from build123d import *

# Parameters (mm, degrees)
SKETCH_190_W        = 36
SKETCH_190_H        = 26.8
EXTRUDE_1_DEPTH     = 16.5
SKETCH_353_W        = 34
SKETCH_353_H        = 24.8
CUT_EXTRUDE_1_DEPTH = 14.5
SKETCH_4_W          = 23.5
SKETCH_4_H          = 23.5
CUT_EXTRUDE_2_DEPTH = 1
SKETCH_5_R          = 11.7
CUT_EXTRUDE_3_DEPTH = 6
SKETCH_11_W         = 2.5
SKETCH_11_H         = 1
CUT_EXTRUDE_6_DEPTH = 2


with BuildPart() as part:
    # Sketch 190 → 凸台-拉伸1 (new body)
    with BuildSketch(Plane(origin=(0, 0, 0), x_dir=(1, 0, 0), z_dir=(0, 1, 0))):
        Rectangle(SKETCH_190_W, SKETCH_190_H)
    extrude(amount=EXTRUDE_1_DEPTH)

    # Sketch 353 → 切除-拉伸1 (cut)
    with BuildSketch(Plane(origin=(0, 0, 0), x_dir=(-1, 0, 0), z_dir=(0, -1, 0))):
        Rectangle(SKETCH_353_W, SKETCH_353_H)
    extrude(amount=-CUT_EXTRUDE_1_DEPTH, mode=Mode.SUBTRACT)

    # 草图4 → 切除-拉伸2 (cut)
    with BuildSketch(Plane.XZ.offset(-14.5)):
        Rectangle(SKETCH_4_W, SKETCH_4_H)
    extrude(amount=-CUT_EXTRUDE_2_DEPTH, mode=Mode.SUBTRACT)

    # 草图5 → 切除-拉伸3 (cut)
    with BuildSketch(Plane.XZ.offset(-15.5)):
        Circle(SKETCH_5_R)
    extrude(amount=-CUT_EXTRUDE_3_DEPTH, mode=Mode.SUBTRACT)

    # 草图11 → 切除-拉伸6 (cut)
    with BuildSketch(Plane(origin=(0, 0, 0), x_dir=(-1, 0, 0), z_dir=(0, -1, 0))):
        with Locations((0, -12.9)):
            Rectangle(SKETCH_11_W, SKETCH_11_H)
    extrude(amount=-CUT_EXTRUDE_6_DEPTH, mode=Mode.SUBTRACT)


solid = part.part
Design review of the part built by this model. Coordinates are the model's own, in mm. A direction names the side the tool comes from. Give positions to 0.01 mm unless a question says otherwise; leave off trailing zeros. Order: outer loops, then holes, each group sorted by start corner. A loop starts at its lowest first (then second) coordinate and runs counter-clockwise, first axis right, second up. Notation, with made-up numbers: (14, -4) - (44, -4) arc R22 cw to (44, 19) - close; hole circle Ø9 at (30.5, -34.75). An arc over 180 degrees is marked (long way). Use CSV: the item, a comma, the result in double quotes. Start each with the question number.
Q1. For line 1 (Z direction, x = 0, y = 16.1); line 2 (X direction, y = 13.5, z = -7.5); line 3 (Z direction, x = -5.5, y = 3.25), list the stretches that pass through material, from the lowest coordinate up.
Q2. Take a section at C-C (y = 2.75). State the section outline as (x, z) points.
Q3. Take a section at A-A (x = 0). State the section outline as (y, z) points.
Q4. Machinability: for faces 4 (the face through (0, 15, -11.75)), 5 (the face through (-1.25, 1, 13)), 6 (the face through (0, 16.5, -12)), which of the approach directions +Z, -Z, +X, -X, +Y, -Y give a long, thin tool a straight path to every point of the face, cutting with its end or side? Answer none if there is none.
Q5. Take a section at B-B (z = 0). State the section outline as (x, y) points, and give its area (3 significant figures).
Q6. Take a section at D-D (x = 13). State the section outline as (y, z) points.
Q7. Draft analysis for pull direction X (two halves, no side actions). For faces 1 (the face through (0, 0, -13)), 2 (the face through (18, 8, 0)), 3 (the face through (0, 2, 13)), state which applies: pulls with the +X half, pulls with the -X half, needs draft (parallel to the pull), parting line crosses it, or undercut.
Q8. For P1, Ø1.5, axis at x = -13, z = 4.5, coming from the -Y side; P2, Ø5, axis at x = 6.5, z = -3.5, coming from the -Y side, all flat-tipped, find the tip position at first contact; note any pin that passes through.
Calculated:
1,line 1,"z = -13.4 to -11.7, 11.7 to 13.4"
1,line 2,"x = -18 to -17, 17 to 18"
1,line 3,"z = -13.4 to -12.4, 12.4 to 13.4"
2,outline,"(-18, -13.4) - (18, -13.4) - (18, 13.4) - (-18, 13.4) - close; hole (-17, -12.4) - (17, -12.4) - (17, 12.4) - (-17, 12.4) - close"
3,outline,"(0, -13.4) - (16.5, -13.4) - (16.5, -11.7) - (15.5, -11.7) - (15.5, -11.75) - (14.5, -11.75) - (14.5, -12.4) - (0, -12.4) - close; (2, 12.4) - (14.5, 12.4) - (14.5, 11.75) - (15.5, 11.75) - (15.5, 11.7) - (16.5, 11.7) - (16.5, 13.4) - (2, 13.4) - close"
4,face 4,"-Y"
4,face 5,"+Z, -Y"
4,face 6,"+Z, -Z, +X, -X, +Y"
5,outline,"(-18, 0) - (-17, 0) - (-17, 14.5) - (-11.75, 14.5) - (-11.75, 15.5) - (-11.7, 15.5) - (-11.7, 16.5) - (-18, 16.5) - close; (11.7, 15.5) - (11.75, 15.5) - (11.75, 14.5) - (17, 14.5) - (17, 0) - (18, 0) - (18, 16.5) - (11.7, 16.5) - close"
5,area,"54.1 mm²"
6,outline,"(0, -13.4) - (16.5, -13.4) - (16.5, 13.4) - (0, 13.4) - (0, 12.4) - (14.5, 12.4) - (14.5, -12.4) - (0, -12.4) - close"
7,face 1,"needs draft"
7,face 2,"pulls with the +X half"
7,face 3,"undercut"
8,P1,"stops at y = 14.5"
8,P2,"passes through"
